Could you check a few things on this model? Use its own coordinates, in mm. Face numbers are marked on the shaded views. A direction names the side the tool comes from. Give positions to 0.01 mm unless a question says otherwise; leave off trailing zeros. Order: outer loops, then holes, each group sorted by start corner. A loop starts at its lowest first (then second) coordinate and runs counter-clockwise, first axis right, second up. Notation, with made-up numbers: (8, -34) -> (42, -34) arc R19 ccw to (42, 2) -> close; hole circle Ø1 at (-11.75, 27.5). An arc over 180 degrees is marked (long way). One line per item, written item: value.
```python
from build123d import *

# Parameters (mm, degrees)
F0_R     = 8
F1_DEPTH = 1
F2_R     = 6
F3_DEPTH = 10
F5_DEPTH = 7
F6_SIZE  = 1
F8_R     = 6
F8_R_2   = 5.5070026954
F9_DEPTH = 9


with BuildPart() as f1:
    # F0 (on Top) → F1 (new body)
    with BuildSketch(Plane.XY):
        Circle(F0_R)
    extrude(amount=F1_DEPTH)

    # F2 (on face) → F3 (join)
    with BuildSketch(Plane(origin=(0, 0, 0), x_dir=(1, 0, 0), z_dir=(0, 0, -1))):
        Circle(F2_R)
    extrude(amount=F3_DEPTH)

    # F4 (on face) → F5 (cut)
    with BuildSketch(Plane(origin=(0, 0, -10), x_dir=(1, 0, 0), z_dir=(0, 0, -1))):
        with BuildLine():
            ThreePointArc((5.8094750193, -1.5), (5.9521781776, -0.7560257549), (6, 0))
            ThreePointArc((6, 0), (5.9521781776, 0.7560257549), (5.8094750193, 1.5))
            Line((5.8094750193, 1.5), (-5.8094750193, 1.5))
            ThreePointArc((-5.8094750193, 1.5), (-6, 0), (-5.8094750193, -1.5))
            Line((-5.8094750193, -1.5), (5.8094750193, -1.5))
        make_face()
    extrude(amount=-F5_DEPTH, mode=Mode.SUBTRACT)

    # F6
    f6_edges = [f1.edges().sort_by_distance(p)[0] for p in [
        (0, 6, -10),
        (0, -6, -10),
    ]]
    chamfer(f6_edges, length=F6_SIZE)

    # F8 (on offset) → F9 (cut)
    with BuildSketch(Plane(origin=(0, 0, -9), x_dir=(1, 0, 0), z_dir=(0, 0, -1))):
        Circle(F8_R)
        Circle(F8_R_2, mode=Mode.SUBTRACT)
    extrude(amount=-F9_DEPTH, mode=Mode.SUBTRACT)


solid = f1.part
```
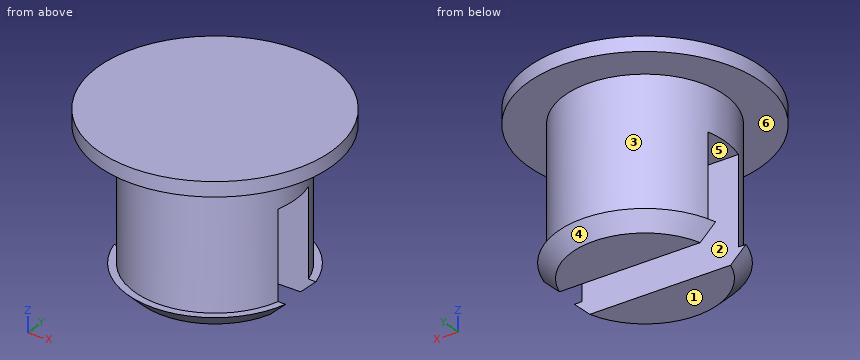
1) For the marked faces 4, 5 and 6, which set-ups out of +Z, -Z, +X, -X, +Y, -Y let a thin tool reach every point of the face, with its end or its side?
Answer below:
face 4: -Z, +Y
face 5: -Z, +X, -X
face 6: none
2) Suppose I cut it at B-B, the plane y = 0. Write out the boundary of the cut face in (x, z).
Answer below:
outline: (-8, 0) -> (-5.51, 0) -> (-5.51, -3) -> (5.51, -3) -> (5.51, 0) -> (8, 0) -> (8, 1) -> (-8, 1) -> close
3) We'd pull the mould along Z, two halves only. Please class the marked faces 1, 2 and 3: +Z half, -Z half, draft (parallel to the pull), parting line (faces both ways), or undercut.
Answer below:
face 1: -Z half
face 2: draft
face 3: undercut
4) For P1, Ø6, axis at y = 2, z = -4, coming from the +X side; P2, Ø3, axis at y = 5, z = -6.5, coming from the -X side; P3, Ø4, axis at x = 3.5, z = -5.5, coming from the -Y side; P4, Ø6, axis at x = 4.5, y = 0, coming from the -Z side, each with a flat end and sliding along its axis, tell me the tip position at first contact or that it passes through.
Answer below:
P1: stops at x = 5.51
P2: stops at x = -4.25
P3: stops at y = -5.3
P4: stops at z = -10
5) Suppose I cut it at A-A, the plane x = 0. Write out the boundary of the cut face in (y, z), then the cut area to 3 significant figures.
Answer below:
outline: (-8, 0) -> (-5.51, 0) -> (-5.51, -9) -> (-6, -9) -> (-5, -10) -> (-1.5, -10) -> (-1.5, -3) -> (1.5, -3) -> (1.5, -10) -> (5, -10) -> (6, -9) -> (5.51, -9) -> (5.51, 0) -> (8, 0) -> (8, 1) -> (-8, 1) -> close
area: 105 mm2
6) If I drill on line 1 along Y through (x, z) = (-2.75, -4.75); line 2 along Z through (x, y) = (1.75, 0.25); line 3 along Z through (x, y) = (5.25, -5.5), over which ranges is the centre line in solid material (lowest first)?
Answer below:
line 1: y = -4.77 to -1.5, 1.5 to 4.77
line 2: z = -3 to 1
line 3: z = 0 to 1
7) Suppose I cut it at C-C, the plane z = -6.75. Write out the boundary of the cut face in (x, y).
Answer below:
outline: (-5.3, -1.5) arc R5.51 ccw to (5.3, -1.5) -> close; (-5.3, 1.5) -> (5.3, 1.5) arc R5.51 ccw to start
8) Suppose I cut it at D-D, the plane z = -2.5. Write out the boundary of the cut face in (x, y), then the cut area to 3 significant figures.
Answer below:
outline: circle Ø11.01 at (0, 0)
area: 95.3 mm2
